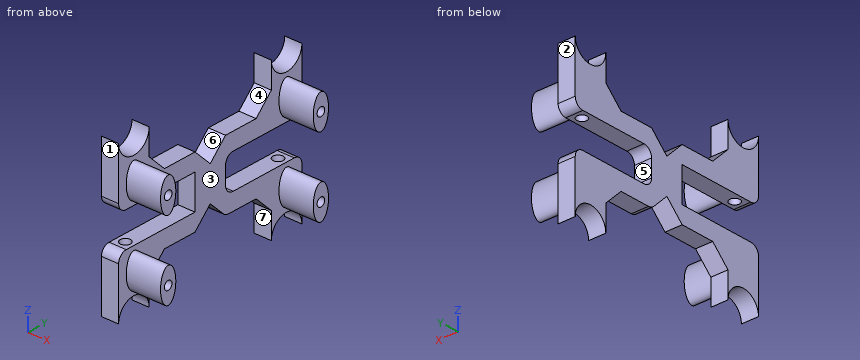
from build123d import *

# Parameters (mm, degrees)
BOSS_EXTRUDE1_DEPTH = 20
SKETCH1_4_RX        = 20
SKETCH1_4_RY        = 10
SKETCH1_4_R         = 5
BOSS_EXTRUDE2_DEPTH = 40
SKETCH2_R           = 6
CUT_EXTRUDE1_DEPTH  = 35
FILLET1_R           = 10


with BuildPart() as part:
    # Sketch1 → Boss-Extrude1 (new body)
    with BuildSketch(Plane(origin=(0, 0, 0), x_dir=(0, 0, -1), z_dir=(1, 0, 0))):
        with BuildLine():
            Line((0, 0), (0, 20))
            Line((0, 20), (20, 20))
            Line((20, 20), (20, 110))
            ThreePointArc((20, 110), (22.928932188, 117.071067812), (30, 120))
            Line((30, 120), (90, 120))
            ThreePointArc((90, 120), (70, 100), (90, 80))
            Line((90, 80), (60, 80))
            Line((60, 80), (40, 60))
            Line((40, 60), (40, 20))
            Line((40, 20), (20, 0))
            Line((20, 0), (0, 0))
        make_face()
    extrude(amount=-BOSS_EXTRUDE1_DEPTH)

    # Sketch1<4> → Boss-Extrude2 (add)
    with BuildSketch(Plane(origin=(0, 0, 0), x_dir=(0, 0, -1), z_dir=(1, 0, 0))):
        with Locations(Location((45, 100), (0, 0, 180))):
            Ellipse(SKETCH1_4_RX, SKETCH1_4_RY)
        with Locations((45, 100)):
            Circle(SKETCH1_4_R, mode=Mode.SUBTRACT)
    extrude(amount=BOSS_EXTRUDE2_DEPTH)

    # Sketch2 → Cut-Extrude1 (cut)
    with BuildSketch(Plane.XY.offset(-20)):
        with Locations((-10, 100)):
            Circle(SKETCH2_R)
    extrude(amount=-CUT_EXTRUDE1_DEPTH, mode=Mode.SUBTRACT)

    # Mirror1: part across plane


with BuildPart() as part_1:
    add(part.part)
    add(part.part.mirror(Plane(origin=(-20, 0, 0), x_dir=(1, 0, 0), z_dir=(0, 0, -1))))

    # Mirror2: part across plane


with BuildPart() as part_2:
    add(part_1.part)
    add(part_1.part.mirror(Plane(origin=(-20, 0, -20), x_dir=(0, 0, 1), z_dir=(0, 1, 0))))

    # Fillet1
    fillet1_edges = [part_2.edges().sort_by_distance(p)[0] for p in [
        (-10, 20, -40),
        (-10, 20, -20),
        (-10, 20, 20),
    ]]
    fillet(fillet1_edges, radius=FILLET1_R)


solid = part_2.part
Source: CAD feature listing. Evaluate the final solid. Frame: model axes, mm. Face numbers are marked on the shaded views. A direction names the side the tool comes from. Give positions to 0.01 mm unless a question says otherwise; leave off trailing zeros. Order: outer loops, then holes, each group sorted by start corner. A loop starts at its lowest first (then second) coordinate and runs counter-clockwise, first axis right, second up. Notation, with made-up numbers: (41.5, -17) -> (79.5, -17) arc R25 ccw to (79.5, 3) -> close; hole circle Ø1 at (-6.5, -15). An arc over 180 degrees is marked (long way). Write item = value, one per line.
Item 1: Contact query for flat-ended pins moving along their axis: pin 1 (2 mm diameter, centred on x = 12.5, z = 40, fed in from +Y); pin 2 (9.5 mm diameter, centred on x = -10, y = 100, fed in from +Z); pin 3 (6 mm diameter, centred on x = -14.5, y = -44.5, fed in from -Z). Output: stop coordinate, or through.
Check result:
pin_1 = 109.8
pin_2 = 70.57
pin_3 = -40
Item 2: Ray query, probe 1 along Y at (x, z) = (29, 45); probe 2 along Y at (x, z) = (-10, 30); probe 3 along X at (y, z) = (-100, 30). Return the intervals inside material, ascending.
Check result:
probe_1 = -110 to -105, -95 to -90, 90 to 95, 105 to 110
probe_2 = -120 to -106, -94 to -10, 10 to 94, 106 to 120
probe_3 = -20 to -16, -4 to 40
Item 3: Section query B-B (x = 30). State how many separate pieces and enclosed holes the cut face has, then the cut area to 3 significant figures.
Check result:
separate_pieces = 4
enclosed_holes = 4
area = 2,200 mm²
Item 4: Section query A-A (y = 54). Output: boundary loops of the cut face in (x, z).
Check result:
outline = (-20, -40) -> (0, -40) -> (0, -20) -> (-20, -20) -> close; (-20, 20) -> (0, 20) -> (0, 40) -> (-20, 40) -> close
Item 5: Set-up query: the marked faces 5, 6 and 7. Return all of +Z, -Z, +X, -X, +Y, -Y with unobstructed straight access to the full face (end or side cutting, diameter ignored); none if empty.
Check result:
face_5 = +X, -X, +Y
face_6 = +Z, +X, -X
face_7 = -Z, +X, -X
Item 6: Section query D-D (z = -3). Output: boundary loops of the cut face in (x, y).
Check result:
outline = (-20, -20) -> (0, -20) -> (0, 20) -> (-20, 20) -> close
Item 7: Mould query, pull axis Y, two halves, no side actions, for the marked faces 1, 2, 3 and 4. Classes: +Y half, -Y half, draft (parallel to the pull), parting line (faces both ways), or undercut.
Check result:
face_1 = -Y half
face_2 = +Y half
face_3 = undercut
face_4 = undercut
